Work out the finished part from the listing and answer in its coordinate system (mm). A direction names the side the tool comes from. Round coordinates to 2 decimals unless told otherwise and drop trailing zeros. Order: outer loops, then holes, each group sorted by start corner. A loop starts at its lowest first (then second) coordinate and runs counter-clockwise, first axis right, second up. Notation, with made-up numbers: (7, 33) - (59, 33) arc R22 cw to (59, 66) - close; hole circle Ø5 at (32, 68.25). An arc over 180 degrees is marked (long way). Put each result on its own line as item: value.
Autodesk Fusion 360 part; units mm, degrees
sketch "Skizze7" plane through (0, 0, 0) normal (0, 0, 1) x (1, 0, 0)
  line L0 (40, 0) -> (40, 56)
  line L1 (0, 0) -> (40, 0)
  line L2 (0, 56) -> (0, 0)
  line L3 (40, 56) -> (0, 56)
  line L4 (19.1939, 4.7) -> (20.8061, 4.7)
  line L5 (20.8061, 1.3) -> (19.1939, 1.3)
  line L6 (24.4922, 4.7) -> (24.4922, 1.3)
  line L7 (15.5, 1.3) -> (15.5, 4.7)
  line L8 (30.4001, 18.6999) -> (9.5999, 18.6999)
  line L9 (30.4001, 16.2998) -> (30.4001, 18.6999)
  line L10 (9.5999, 18.6999) -> (9.5999, 16.2998)
  line L11 (9.5999, 16.2998) -> (30.4001, 16.2998)
  circle A0 centre (34, 18) radius 1.6
  circle A1 centre (6, 18) radius 1.6
  line L12 (15.5, 3) -> (24.4922, 3) construction
  line L13 (20, 4.7) -> (20, 1.3) construction
  line L14 (16.9808, 1.5) -> (23.0114, 1.5)
  arc A2 (23.0114, 1.5) -> (23.0114, 4.5) centre (23.0114, 3) ccw
  line L15 (23.0114, 4.5) -> (16.9808, 4.5)
  arc A3 (16.9808, 4.5) -> (16.9808, 1.5) centre (16.9808, 3) ccw
  line L16 (16.9808, 3) -> (23.0114, 3) construction
  point P0 (19.9961, 3)
  dimension "d25" = 3
extrude "Extrusion10" add sketch "Skizze7" along normal blind 1.6 contours L0 L1 L2 L3 | L6 L7 L14 A2 L15 A3 | L8 L9 L10 L11
extrude "Extrusion11" add sketch "Skizze7" against normal blind 9.3 contours L6 L7 L14 A2 L15 A3
sketch "Skizze8" plane through (0, 0, 1.6) normal (0, 0, 1) x (-1, 0, 0)
  line L0 (-15.5, -3.2394) -> (-15.5, -2.7606)
  arc A0 (-15.5, -3.2394) -> (-15.5, -2.7606) centre (-16.9808, -3) ccw
  circle A1 centre (-6, -18) radius 1.6
  line L1 (-24.4922, -2.7606) -> (-24.4922, -3.2394)
  arc A2 (-24.4922, -2.7606) -> (-24.4922, -3.2394) centre (-23.0114, -3) ccw
  circle A3 centre (-34, -18) radius 1.6
  line L2 (-40, -56) -> (0, -56)
  line L3 (0, -56) -> (0, 0)
  line L4 (0, 0) -> (-40, 0)
  line L5 (-40, 0) -> (-40, -56)
  line L6 (-9.5999, -16.2998) -> (-30.4001, -16.2998)
  line L7 (-30.4001, -18.6999) -> (-9.5999, -18.6999)
  line L8 (-30.4001, -16.2998) -> (-30.4001, -18.6999)
  line L9 (-9.5999, -18.6999) -> (-9.5999, -16.2998)
extrude "Extrusion12" add sketch "Skizze8" along normal blind 8.3 contours L6 L7 L8 L9
sketch "Skizze9" plane through (0, 0, 9.9) normal (0, 0, 1) x (-1, 0, 0)
  line L0 (-9.5999, -18.6999) -> (-9.5999, -16.2998)
  line L1 (-9.5999, -16.2998) -> (-30.4001, -16.2998)
  line L2 (-30.4001, -16.2998) -> (-30.4001, -18.6999)
  line L3 (-30.4001, -18.6999) -> (-9.5999, -18.6999)
  line L4 (-30.4001, -17.4999) -> (-9.5999, -17.4999) construction
  circle A0 centre (-28.89, -17.4999) radius 0.45
  circle A1 centre (-26.35, -17.4999) radius 0.45
  circle A2 centre (-23.81, -17.4999) radius 0.45
  circle A3 centre (-21.27, -17.4999) radius 0.45
  circle A4 centre (-18.73, -17.4999) radius 0.45
  circle A5 centre (-16.19, -17.4999) radius 0.45
  circle A6 centre (-13.65, -17.4999) radius 0.45
  circle A7 centre (-11.11, -17.4999) radius 0.45
  dimension "d32" = 0.9
  dimension "d35" = 2.54
  dimension "d36" = 0
  dimension "d37" = 1.5101
  dimension "d38" = 1.5101
extrude "Extrusion13" cut sketch "Skizze9" against normal up to surface (8.3 mm away) contours A0 | A1 | A2 | A3 | A4 | A5 | A6 | A7
equation "d37 = d38"
1) A cutting plane is placed at B-B on z = 2.75. Give the number of separate pieces and of enclosed holes in the cut face, then the cut area to 3 significant figures.
Findings below:
separate pieces: 1
enclosed holes: 8
area: 44.8 mm2
2) Straight lines are drawn through the part: L1, parallel to Y at x = 34, z = 1.1; L2, parallel to Y at x = 28.89, z = 5.25; L3, parallel to Z at x = 6.5, y = 29.5. For each, find the intervals that lie inside material, in ascending order. Write a range as from..to.
Findings below:
L1: y = 0..16.4, 19.6..56
L2: y = 16.3..17.05, 17.95..18.7
L3: z = 0..1.6
3) A cutting plane is placed at D-D on y = 41.5. Write down the section's boundary in (x, z).
Findings below:
outline: (0, 0) - (40, 0) - (40, 1.6) - (0, 1.6) - close
4) A cutting plane is placed at A-A on x = 6. Write down the section's boundary in (y, z), then the cut area to 3 significant figures.
Findings below:
outline: (0, 0) - (16.4, 0) - (16.4, 1.6) - (0, 1.6) - close; (19.6, 0) - (56, 0) - (56, 1.6) - (19.6, 1.6) - close
area: 84.5 mm2
5) Given pin 1 Ø4 at (x, y) = (6, 18) entering from -Z; pin 2 Ø0.7 at (y, z) = (17.5, 7) entering from -X; pin 3 Ø3.5 at (x, y) = (34, 18) entering from +Z; pin 4 Ø5 at (x, z) = (33.5, -3.5) entering from -Y, each flat-ended and moving along its own axis, determine where each tip first touches the part or whether it passes through.
Findings below:
pin 1: stops at z = 0
pin 2: stops at x = 9.6
pin 3: stops at z = 1.6
pin 4: passes through
6) A cutting plane is placed at C-C on z = -6.5. Write down the section's boundary in (x, y), then the cut area to 3 significant figures.
Findings below:
outline: (15.5, 2.76) arc R1.5 ccw to (16.98, 1.5) - (23.01, 1.5) arc R1.5 ccw to (24.49, 2.76) - (24.49, 3.24) arc R1.5 ccw to (23.01, 4.5) - (16.98, 4.5) arc R1.5 ccw to (15.5, 3.24) - close
area: 25.1 mm2
7) For a pull along Y with two mould halves and no side action, classify faces 1 (the flat face through (20, 28, 1.6)), 2 (the cylindrical face through (32.82, 16.92, 0.79)), 3 (the cylindrical face through (24, 4.13, -4.58)) as pulls with the +Y half, pulls with the -Y half, needs draft (parallel to the pull), parting line crosses it, or undercut.
Findings below:
face 1: needs draft
face 2: undercut
face 3: pulls with the +Y half
8) For faces 4 (the flat face through (20, 18.7, 6)), 5 (the flat face through (30.4, 17, 6)), 6 (the cylindrical face through (15.997, 1.868, -4.585)), 7 (the cylindrical face through (23.972, 1.848, -4.585)), determine the directions among +Z, -Z, +X, -X, +Y, -Y from which every point of the face is accessible in a straight line to the end or side of a thin tool.
Findings below:
face 4: +Z, +X, -X, +Y
face 5: +Z, +X, +Y, -Y
face 6: -Z, -X, -Y
face 7: -Z, +X, -Y
